```python
from build123d import *

# Parameters (mm, degrees)
EXTRUDE_1_DEPTH = 10
EXTRUDE_2_DEPTH = 20
FILLET_1_R      = 5


with BuildPart() as part:
    # Sketch 1 → Extrude 1 (new body)
    with BuildSketch(Plane(origin=(0, 0, 0), x_dir=(1, 0, 0), z_dir=(0, 1, 0))):
        with BuildLine():
            Line((-7.5, 5), (-7.5, -10))
            Line((-7.5, -10), (2.5, -10))
            Line((2.5, -10), (2.5, -5))
            ThreePointArc((2.5, -5), (3.964466094, -1.464466094), (7.5, 0))
            Line((7.5, 0), (12.5, 0))
            Line((12.5, 0), (12.5, 5))
            Line((12.5, 5), (-7.5, 5))
        make_face()
        Polygon((-12.5, 5), (-12.5, -10), (-7.5, -10), (-7.5, 5), (12.5, 5), (12.5, 10), (-7.5, 10), (-12.5, 10), align=None)
    extrude(amount=EXTRUDE_1_DEPTH)

    # Sketch 1_3 → Extrude 2 (add)
    with BuildSketch(Plane(origin=(0, 0, 0), x_dir=(1, 0, 0), z_dir=(0, 1, 0))):
        Polygon((-12.5, 5), (-12.5, -10), (-7.5, -10), (-7.5, 5), (12.5, 5), (12.5, 10), (-7.5, 10), (-12.5, 10), align=None)
    extrude(amount=EXTRUDE_2_DEPTH)

    # Fillet 1
    fillet_1_edges = [part.edges().sort_by_distance(p)[0] for p in [
        (12.5, 20, -7.5),
        (-10, 20, 10),
    ]]
    fillet(fillet_1_edges, radius=FILLET_1_R)


solid = part.part
```
Part model, mm, in its own coordinate system. A direction names the side the tool comes from. Round coordinates to 2 decimals unless told otherwise and drop trailing zeros. Loops run counter-clockwise (first coordinate to the right, second up) from the corner with the lowest first, then second, coordinate; pieces in that order, holes last.
Item 1: 3-axis set-ups, long thin cutter, end or side, ignore diameter. For faces 1 (the face through (-7.5, 15, 3)), 2 (the face through (11.07, 18.5, -7.54)), 3 (the face through (2.5, 5, 8)): which of +Z, -Z, +X, -X, +Y, -Y reach the whole face in a straight line?
Item 2: Drill centre lines: line 1 (X direction, y = 17, z = 0); line 2 (Y direction, x = 0.5, z = 2.25); line 3 (Z direction, x = 3, y = 15.25). Where is each one in solid material? Low to high.
Item 3: Drop flat-ended pins along their axis: P1, Ø11, axis at y = 16.5, z = -0.5, coming from the +X side; P2, Ø5.5, axis at y = 2.5, z = 7, coming from the +X side; P3, Ø2, axis at x = 10, y = 5, coming from the +Z side; P4, Ø3, axis at x = 8.5, z = 3, coming from the +Y side. Give the stop position or say it passes through.
Item 4: Cut at C-C, the plane z = -2.5. Give the cut face in (x, y), then the cut area to 3 significant figures.
Item 5: Cut at B-B, the plane x = 4.5. Give the cut face in (y, z), then the cut area to 3 significant figures.
Item 6: Cut at A-A, the plane y = 6.5. Give the cut face in (x, z).
A:
1. face 1: +Z, +X, +Y
1. face 2: +Z, -Z, +X, +Y
1. face 3: +Z, +X, +Y, -Y
2. line 1: x = -12.5 to -7.5
2. line 2: y = 0 to 10
2. line 3: z = -10 to -5
3. P1: stops at x = 12.5
3. P2: stops at x = 2.56
3. P3: stops at z = 0
3. P4: passes through
4. outline: (-12.5, 0) - (12.5, 0) - (12.5, 10) - (-7.5, 10) - (-7.5, 20) - (-12.5, 20) - close
4. area: 300 mm2
5. outline: (0, -10) - (20, -10) - (20, -5) - (10, -5) - (10, 1) - (0, 1) - close
5. area: 160 mm2
6. outline: (-12.5, -10) - (12.5, -10) - (12.5, 0) - (7.5, 0) arc R5 cw to (2.5, 5) - (2.5, 10) - (-12.5, 10) - close
